Read the model definition and answer for the solid it produces. Units are mm, in the model's axes. Round coordinates to 2 decimals unless told otherwise and drop trailing zeros. Loops run counter-clockwise (first coordinate to the right, second up) from the corner with the lowest first, then second, coordinate; pieces in that order, holes last. Notation, with made-up numbers: (-13.5, 16.25) -> (37.5, 16.25) arc R12 cw to (37.5, 36.25) -> close; hole circle Ø7 at (42, 30). An arc over 180 degrees is marked (long way). Put each result on its own line as item: value.
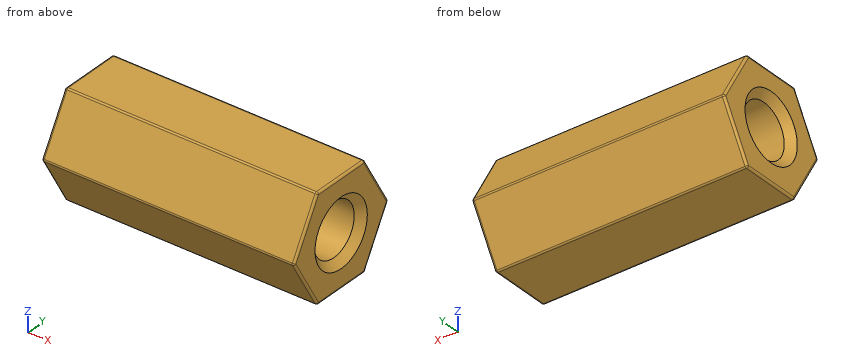
from build123d import *

# Parameters (mm, degrees)
BOSS_EXTRUDE1_DEPTH = 12
FILLET1_R           = 0.1


with BuildPart() as part:
    # Sketch1 → Boss-Extrude1 (new body)
    with BuildSketch(Plane(origin=(12, 0, 0), x_dir=(0, 0, -1), z_dir=(1, 0, 0))):
        Polygon((-2.5, 1.443375673), (-2.5, -1.443375673), (0, -2.886751346), (2.5, -1.443375673), (2.5, 1.443375673), (0, 2.886751346), align=None)
    extrude(amount=-BOSS_EXTRUDE1_DEPTH)

    # Sketch2 → Cut-Revolve1 (revolve, cut)
    with BuildSketch(Plane.XY):
        Polygon((0, 1.6), (0, 0), (12, 0), (12, 1.6), (11.649, 1.25), (0.351, 1.25), (0.001, 1.6), align=None)
    revolve(axis=Axis((0, 0, 0), (1, 0, 0)), mode=Mode.SUBTRACT)

    # Fillet1
    fillet1_edges = [part.edges().sort_by_distance(p)[0] for p in [
        (0, -2.165063509, 1.25),
        (6, 2.886751346, 0),
        (6, 1.443375673, -2.5),
        (6, -1.443375673, -2.5),
        (6, -2.886751346, 0),
        (6, -1.443375673, 2.5),
        (6, 1.443375673, 2.5),
        (0, -2.165063509, -1.25),
        (0, 0, -2.5),
        (0, 2.165063509, -1.25),
        (0, 2.165063509, 1.25),
        (12, 2.165063509, -1.25),
        (12, 0, -2.5),
        (12, -2.165063509, -1.25),
        (0, 0, 2.5),
        (12, -2.165063509, 1.25),
        (12, 0, 2.5),
        (12, 2.165063509, 1.25),
    ]]
    fillet(fillet1_edges, radius=FILLET1_R)


solid = part.part
Item 1: Find the intervals of material crossed by line 1 along Z through (x, y) = (7.5, -0.05); line 2 along Z through (x, y) = (3, 0.6); line 3 along Z through (x, y) = (4.75, 1.5), in increasing order.
Derived:
line 1: z = -2.5 to -1.25, 1.25 to 2.5
line 2: z = -2.5 to -1.1, 1.1 to 2.5
line 3: z = -2.4 to 2.4
Item 2: A flat-ended cylindrical pin translates along its axis: pin 1 Ø2 at (x, z) = (7.5, -1.5) entering from +Y. Find the tip coordinate at first contact, or state that the pin passes through.
Derived:
pin 1: stops at y = 2.6
Item 3: The part is cut by section B-B (x = 8.5). Determine the outline of the cut face in (y, z).
Derived:
outline: (-2.86, -0.05) -> (-1.47, -2.45) arc R0.1 ccw to (-1.39, -2.5) -> (1.39, -2.5) arc R0.1 ccw to (1.47, -2.45) -> (2.86, -0.05) arc R0.1 ccw to (2.86, 0.05) -> (1.47, 2.45) arc R0.1 ccw to (1.39, 2.5) -> (-1.39, 2.5) arc R0.1 ccw to (-1.47, 2.45) -> (-2.86, 0.05) arc R0.1 ccw to start; hole circle Ø2.5 at (0, 0)
